from build123d import *

# Parameters (mm, degrees)
F0_W     = 99.988638
F0_H     = 34.840912
F1_DEPTH = 12
F2_R     = 3
F3_DEPTH = 75


with BuildPart() as f1:
    # F0 (on Front) → F1 (new body)
    with BuildSketch(Plane.XZ):
        with Locations((0.954544, 1.073864)):
            Rectangle(F0_W, F0_H)
    extrude(amount=F1_DEPTH)

    # F2 (on face) → F3 (cut)
    with BuildSketch(Plane(origin=(0, 0, 0), x_dir=(-1, 0, 0), z_dir=(0, 1, 0))):
        with Locations((-28.039774, 0)):
            Circle(F2_R)
        with Locations((28.039774, 0)):
            Circle(F2_R)
    extrude(amount=-F3_DEPTH, mode=Mode.SUBTRACT)


solid = f1.part
Check sheet for the modelled part. Datum: model origin and axes. Units: mm. Round coordinates to 2 decimals unless told otherwise and drop trailing zeros. Order: outer loops, then holes, each group sorted by start corner. A loop starts at its lowest first (then second) coordinate and runs counter-clockwise, first axis right, second up.
(1) Cross-section at B-B, the plane y = -1.25. Enter the section's corners in (x, z), and give its area (3 significant figures).
(2) Go/stop test with a flat-tipped pin: P1, Ø5.5, axis at x = -28.04, z = 0, coming from the -Y side. Record where the tip stops, or that it passes through.
(3) Draft check along Z on faces 1 (the flat face through (0, -6, 18.494)), 2 (the flat face through (0, -6, -16.347)), 3 (the cylindrical face through (25.27, -5.92, -1.15)), 4 (the flat face through (-49.04, -6, 1)). Enter one of: pulls with the +Z half, pulls with the -Z half, needs draft (parallel to the pull), parting line crosses it, or undercut.
(4) Scan lines: probe 1 along X at (y, z) = (-5, -1); probe 2 along X at (y, z) = (-0.75, 0.5). Record each from-to range of solid material in increasing order.
(5) Cross-section at A-A, the plane z = 0. Enter the section's corners in (x, y).
Check sheet entries:
1. outline: (-49.04, -16.35) - (50.95, -16.35) - (50.95, 18.49) - (-49.04, 18.49) - close; hole circle Ø6 at (-28.04, 0); hole circle Ø6 at (28.04, 0)
1. area: 3,430 mm2
2. P1: passes through
3. face 1: pulls with the +Z half
3. face 2: pulls with the -Z half
3. face 3: undercut
3. face 4: needs draft
4. probe 1: x = -49.04 to -30.87, -25.21 to 25.21, 30.87 to 50.95
4. probe 2: x = -49.04 to -31, -25.08 to 25.08, 31 to 50.95
5. outline: (-49.04, -12) - (-31.04, -12) - (-31.04, 0) - (-49.04, 0) - close; (-25.04, -12) - (25.04, -12) - (25.04, 0) - (-25.04, 0) - close; (31.04, -12) - (50.95, -12) - (50.95, 0) - (31.04, 0) - close
